Read the model definition and answer for the solid it produces. Units are mm, in the model's axes. A direction names the side the tool comes from. Round coordinates to 2 decimals unless told otherwise and drop trailing zeros. Loops run counter-clockwise (first coordinate to the right, second up) from the corner with the lowest first, then second, coordinate; pieces in that order, holes last. Notation, with made-up numbers: (42.5, 8.5) - (55.5, 8.5) arc R15 ccw to (55.5, 26.5) - close; hole circle Ø4 at (-1, 2). An arc over 180 degrees is marked (long way). Answer as CSV lines item,"result".
```python
from build123d import *

# Parameters (mm, degrees)
SKETCH_2_W               = 144
SKETCH_2_H               = 240
CUT_EXTRUDE_1_DEPTH      = 15.5
CUT_EXTRUDE_1_DEPTH_BACK = 15.5


with BuildPart() as part:
    # Sketch 1 → Revolve 1 (revolve)
    with BuildSketch(Plane(origin=(0, 0, 0), x_dir=(0, 0, -1), z_dir=(1, 0, 0))):
        with BuildLine():
            Line((-7.75, 8.5), (-7.75, 5))
            Line((-7.75, 5), (6.25, 5))
            Line((6.25, 5), (6.25, 7.2))
            ThreePointArc((6.25, 7.2), (6.2, 7.25), (6.25, 7.3))
            Line((6.25, 7.3), (6.25, 15.75))
            Line((6.25, 15.75), (7.75, 15.75))
            Line((7.75, 15.75), (7.75, 30))
            Line((7.75, 30), (2.25, 30))
            Line((2.25, 30), (2.25, 18))
            Line((2.25, 18), (-3.75, 18))
            Line((-3.75, 18), (-3.75, 15.75))
            Line((-3.75, 15.75), (-1.75, 15.75))
            Line((-1.75, 15.75), (-1.75, 7.25))
            Line((-1.75, 7.25), (-3.75, 7.25))
            Line((-3.75, 7.25), (-3.75, 8.5))
            Line((-3.75, 8.5), (-7.75, 8.5))
        make_face()
    revolve(axis=Axis((0, 0, -7.75), (0, 0, 1)))

    # Sketch 2 → Cut-Extrude 1 (cut, two sides)
    with BuildSketch(Plane.XY) as cut_extrude_1_sk:
        Rectangle(SKETCH_2_W, SKETCH_2_H)
        with BuildLine():
            Line((-12, -13.416408), (-5.457215, -27.883459))
            ThreePointArc((-5.457215, -27.883459), (-4.128934, -29.424934), (-2.17707, -30))
            Line((-2.17707, -30), (2.17707, -30))
            ThreePointArc((2.17707, -30), (4.128934, -29.424934), (5.457215, -27.883459))
            Line((5.457215, -27.883459), (12, -13.416408))
            ThreePointArc((12, -13.416408), (18, 0), (12, 13.416408))
            Line((12, 13.416408), (5.457215, 27.883459))
            ThreePointArc((5.457215, 27.883459), (4.128934, 29.424934), (2.17707, 30))
            Line((2.17707, 30), (-2.17707, 30))
            ThreePointArc((-2.17707, 30), (-4.128934, 29.424934), (-5.457215, 27.883459))
            Line((-5.457215, 27.883459), (-12, 13.416408))
            ThreePointArc((-12, 13.416408), (-18, 0), (-12, -13.416408))
        make_face(mode=Mode.SUBTRACT)
    extrude(amount=CUT_EXTRUDE_1_DEPTH, mode=Mode.SUBTRACT)
    extrude(cut_extrude_1_sk.sketch, amount=-CUT_EXTRUDE_1_DEPTH_BACK, mode=Mode.SUBTRACT)

    # Sketch 3 → Cut-Revolve 1 (revolve, cut)
    with BuildSketch(Plane(origin=(0, 0, 0), x_dir=(0, 0, -1), z_dir=(1, 0, 0))):
        Polygon((-7.75, 22.5), (-7.75, 28.1), (2.25, 28.1), (2.25, 26), (7.75, 26), (7.75, 22.5), align=None)
    revolve(axis=Axis((0, 22.5, -7.75), (0, 0, 1)), mode=Mode.SUBTRACT)

    # Sketch 4 → Cut-Revolve 2 (revolve, cut)
    with BuildSketch(Plane(origin=(0, 0, 0), x_dir=(0, 0, -1), z_dir=(1, 0, 0))):
        Polygon((-7.75, -22.5), (-7.75, -16.9), (2.25, -16.9), (2.25, -19), (7.75, -19), (7.75, -22.5), align=None)
    revolve(axis=Axis((0, -22.5, -7.75), (0, 0, 1)), mode=Mode.SUBTRACT)

    # Sketch 5 → Cut-Revolve 3 (revolve, cut)
    with BuildSketch(Plane(origin=(0, 0, 0), x_dir=(0, 0, -1), z_dir=(1, 0, 0))):
        Polygon((-5.8125, 8.5), (-4.3125, 8.5), (-4.583, 8.2295), (-4.583, 4.9205), (-4.3125, 4.65), (-5.8125, 4.65), align=None)
    revolve(axis=Axis((0, 4.65, 5.8125), (0, 1, 0)), mode=Mode.SUBTRACT)

    # Sketch 6 → Cut-Revolve 4 (revolve, cut)
    with BuildSketch(Plane.XY.offset(5.8125)):
        Polygon((-4.027018, -2.325), (-3.277018, -3.624038), (-3.646528, -3.525028), (-6.512206, -5.179528), (-6.611216, -5.549038), (-7.361216, -4.25), align=None)
    revolve(axis=Axis((-7.361216, -4.25, 5.8125), (0.866025, 0.5, 0)), mode=Mode.SUBTRACT)


solid = part.part
```
1) A cutting plane is placed at B-B, the plane z = -4. Determine the outline of the cut face in (x, y).
Entries:
outline,"(-12, -13.42) - (-5.46, -27.88) arc R3.6 ccw to (-3.31, -29.82) arc R30 ccw to (3.31, -29.82) arc R3.6 ccw to (5.46, -27.88) - (12, -13.42) arc R18 ccw to (12, 13.42) - (5.46, 27.88) arc R3.6 ccw to (3.31, 29.82) arc R30 ccw to (-3.31, 29.82) arc R3.6 ccw to (-5.46, 27.88) - (-12, 13.42) arc R18 ccw to start; hole circle Ø10 at (0, 0); hole circle Ø7 at (0, -22.5); hole circle Ø7 at (0, 22.5)"
2) A cutting plane is placed at D-D, the plane z = -1.25. Determine the outline of the cut face in (x, y), plus the area to 3 significant figures.
Entries:
outline,"(-2.97, -17.75) arc R5.6 cw to (2.97, -17.75) arc R18 ccw to (2.97, 17.75) arc R5.6 cw to (-2.97, 17.75) arc R18 ccw to start; hole circle Ø10 at (0, 0)"
area,"931 mm^2"
3) Find the intervals of material crossed by line 1 (X direction, y = 0, z = 2.9); line 2 (Y direction, x = 0, z = 2.6); line 3 (Y direction, x = -0.5, z = -6), in increasing order.
Entries:
line 1,"x = -18 to -15.75, -7.25 to -5, 5 to 7.25, 15.75 to 18"
line 2,"y = -16.9 to -15.75, -7.25 to -5, 5 to 7.25, 15.75 to 16.9"
line 3,"y = -30 to -25.96, -19.04 to -4.97, 4.97 to 19.04, 25.96 to 30"
4) The mould has two halves that part along X. Classify faces 6 (the face through (0, 30, -5)), 7 (the face through (-1, 16, -7.75)), 8 (the face through (-5, 2, -6.25)): pulls with the +X half, pulls with the -X half, needs draft (parallel to the pull), parting line crosses it, or undercut.
Entries:
face 6,"parting line crosses it"
face 7,"needs draft"
face 8,"undercut"
5) A cutting plane is placed at C-C, the plane x = 15. Determine the outline of the cut face in (y, z).
Entries:
outline,"(-9.95, -7.75) - (-4.8, -7.75) - (-4.8, -6.25) - (4.8, -6.25) - (4.8, -7.75) - (9.95, -7.75) - (9.95, 3.75) - (4.8, 3.75) - (4.8, 1.75) - (-4.8, 1.75) - (-4.8, 3.75) - (-9.95, 3.75) - close"
6) A cutting plane is placed at A-A, the plane y = 0. Determine the outline of the cut face in (x, z).
Entries:
outline,"(-18, -7.75) - (-15.75, -7.75) - (-15.75, -6.25) - (-7.3, -6.25) arc R0.05 cw to (-7.2, -6.25) - (-5, -6.25) - (-5, 7.75) - (-8.5, 7.75) - (-8.5, 3.75) - (-7.25, 3.75) - (-7.25, 1.75) - (-15.75, 1.75) - (-15.75, 3.75) - (-18, 3.75) - close; (5, -6.25) - (7.2, -6.25) arc R0.05 cw to (7.3, -6.25) - (15.75, -6.25) - (15.75, -7.75) - (18, -7.75) - (18, 3.75) - (15.75, 3.75) - (15.75, 1.75) - (7.25, 1.75) - (7.25, 3.75) - (8.5, 3.75) - (8.5, 7.75) - (5, 7.75) - close"
7) Each of these flat-tipped pins is pushed along its axis until it touches: P1, Ø10, axis at x = 12.5, y = 4.5, coming from the +Z side; P2, Ø2, axis at y = 14.5, z = -4, coming from the +X side; P3, Ø1.5, axis at x = 0, z = 5.81, coming from the -Y side; P4, Ø2, axis at x = -11, z = -5.5, coming from the +Y side. Where does it stop, or does it pass through?
Entries:
P1,"stops at z = 7.75"
P2,"stops at x = 11.96"
P3,"stops at y = -8.5"
P4,"stops at y = 17.84"
8) A tool of negligible diameter and unlimited length cuts with its end or side. For faces 1 (the face through (-7.167, 4.57, 5.778)), 2 (the face through (6.43, 3.35, 2.76)), 3 (the face through (0, 16.9, 0.7)), 4 (the face through (-15.616, -2.05, -7.01)), 5 (the face through (-0.05, 6.55, 7.04)), from which of +Z, -Z, +X, -X, +Y, -Y can it reach the whole face along a straight path? Write none if from no direction.
Entries:
face 1,"+Z"
face 2,"none"
face 3,"+Z, +Y"
face 4,"-Z"
face 5,"+Y"
